```python
from build123d import *

# Parameters (mm, degrees)
SKETCH1_W                = 25
SKETCH1_H                = 25
BOSS_EXTRUDE1_DEPTH      = 5
SKETCH2_R                = 1.05
CUT_EXTRUDE1_DEPTH       = 5
FILLET1_R                = 2
SKETCH3_W                = 12
SKETCH3_H                = 12
SKETCH3_W_2              = 6
SKETCH3_H_2              = 6
BOSS_EXTRUDE2_DEPTH      = 98.425
SKETCH4_W                = 6
SKETCH4_H                = 6
CUT_EXTRUDE2_DEPTH       = 10
SKETCH5_W                = 12
SKETCH5_H                = 12
BOSS_EXTRUDE3_DEPTH      = 20
CUT_EXTRUDE3_DEPTH       = 20
CUT_EXTRUDE4_DEPTH       = 20
REVOLVE1_ANGLE           = 25
REVOLVE1_OTHER_WAY_ANGLE = 25


with BuildPart() as part:
    # Sketch1 → Boss-Extrude1 (new body)
    with BuildSketch(Plane(origin=(0, 0, 0), x_dir=(1, 0, 0), z_dir=(0, 1, 0))):
        with Locations((12.5, 12.5)):
            Rectangle(SKETCH1_W, SKETCH1_H)
    extrude(amount=BOSS_EXTRUDE1_DEPTH)

    # Sketch2 → Cut-Extrude1 (cut)
    with BuildSketch(Plane(origin=(0, 5, 0), x_dir=(1, 0, 0), z_dir=(0, 1, 0))):
        with Locations(Location((4.5, 4.5, 0), (0, 0, 270))):
            Circle(SKETCH2_R)
        with Locations(Location((20.5, 4.5, 0), (0, 0, 270))):
            Circle(SKETCH2_R)
        with Locations(Location((20.5, 20.5, 0), (0, 0, 270))):
            Circle(SKETCH2_R)
        with Locations(Location((4.5, 20.5, 0), (0, 0, 270))):
            Circle(SKETCH2_R)
    extrude(amount=-CUT_EXTRUDE1_DEPTH, mode=Mode.SUBTRACT)

    # Fillet1
    fillet1_edges = [part.edges().sort_by_distance(p)[0] for p in [
        (0, 2.5, -25),
        (25, 2.5, -25),
        (25, 2.5, 0),
        (0, 2.5, 0),
    ]]
    fillet(fillet1_edges, radius=FILLET1_R)

    # Sketch3 → Boss-Extrude2 (add)
    with BuildSketch(Plane(origin=(0, 5, 0), x_dir=(1, 0, 0), z_dir=(0, 1, 0))):
        with Locations((12.5, 12.5)):
            Rectangle(SKETCH3_W, SKETCH3_H)
        with Locations((12.5, 12.5)):
            Rectangle(SKETCH3_W_2, SKETCH3_H_2, mode=Mode.SUBTRACT)
    extrude(amount=BOSS_EXTRUDE2_DEPTH)

    # Sketch4 → Cut-Extrude2 (cut)
    with BuildSketch(Plane(origin=(0, 0, 0), x_dir=(-1, 0, 0), z_dir=(0, -1, 0))):
        with Locations((-12.5, 12.5)):
            Rectangle(SKETCH4_W, SKETCH4_H)
    extrude(amount=-CUT_EXTRUDE2_DEPTH, mode=Mode.SUBTRACT)

    # Sketch5 → Boss-Extrude3 (add)
    with BuildSketch(Plane(origin=(0, 103.425, 0), x_dir=(1, 0, 0), z_dir=(0, 1, 0))):
        with Locations((12.5, 12.5)):
            Rectangle(SKETCH5_W, SKETCH5_H)
    extrude(amount=BOSS_EXTRUDE3_DEPTH)

    # Sketch6 → Cut-Extrude3 (cut)
    with BuildSketch(Plane.XY.offset(-6.5)):
        Polygon((18.5, 123.425), (12.5, 123.425), (18.5, 103.425), align=None)
        Polygon((6.5, 103.425), (12.5, 123.425), (6.5, 123.425), align=None)
    extrude(amount=-CUT_EXTRUDE3_DEPTH, mode=Mode.SUBTRACT)

    # Sketch7 → Cut-Extrude4 (cut)
    with BuildSketch(Plane.ZY.offset(-6.5)):
        Polygon((-6.5, 123.425), (-6.5, 103.425), (-12.5, 123.425), align=None)
        Polygon((-18.5, 123.425), (-18.5, 103.425), (-12.5, 123.425), align=None)
    extrude(amount=-CUT_EXTRUDE4_DEPTH, mode=Mode.SUBTRACT)

    # Sketch8 → Revolve1 (revolve)
    with BuildSketch(Plane(origin=(12.5, 0, 0), x_dir=(0, 0, -1), z_dir=(1, 0, 0))):
        with BuildLine():
            ThreePointArc((24.627603923, 50.372343644), (16.394708904, 33.808356072), (20.558863125, 15.785979305))
            Line((20.558863125, 15.785979305), (22.064703847, 16.753815466))
            ThreePointArc((22.064703847, 16.753815466), (18.172495187, 33.599217247), (25.867730183, 49.081471856))
            Line((25.867730183, 49.081471856), (24.627603923, 50.372343644))
        make_face()
    revolve(axis=Axis((12.5, 54.79169199, -43.616981759), (0, -1, 0)), revolution_arc=REVOLVE1_ANGLE)

    # Sketch8 → Revolve1 other way (revolve)
    with BuildSketch(Plane(origin=(12.5, 0, 0), x_dir=(0, 0, -1), z_dir=(1, 0, 0))):
        with BuildLine():
            ThreePointArc((24.627603923, 50.372343644), (16.394708904, 33.808356072), (20.558863125, 15.785979305))
            Line((20.558863125, 15.785979305), (22.064703847, 16.753815466))
            ThreePointArc((22.064703847, 16.753815466), (18.172495187, 33.599217247), (25.867730183, 49.081471856))
            Line((25.867730183, 49.081471856), (24.627603923, 50.372343644))
        make_face()
    revolve(axis=Axis((12.5, 54.79169199, -43.616981759), (0, 1, 0)), revolution_arc=REVOLVE1_OTHER_WAY_ANGLE)


solid = part.part
```
Work out the finished part from the listing and answer in its coordinate system (mm). A direction names the side the tool comes from. Give positions to 0.01 mm unless a question says otherwise; leave off trailing zeros. Write each loop counter-clockwise with the first axis right and the second up, starting at its lowest first coordinate (ties: lowest second). Pieces come first, ordered by that corner, then holes.
(1) Flat-ended cylindrical pins translate along their axes: pin 1 Ø2.5 at (x, y) = (14, 3) entering from -Z; pin 2 Ø5 at (x, y) = (3, 105) entering from +Z; pin 3 Ø5 at (x, z) = (12, -5.5) entering from -Y; pin 4 Ø5 at (y, z) = (76.5, -19.5) entering from -X. Find the tip coordinate at first contact, or state that the pin passes through.
Final values:
pin 1: stops at z = -25
pin 2: passes through
pin 3: stops at y = 0
pin 4: stops at x = 6.5
(2) Which of the six approach directions +Z, -Z, +X, -X, +Y, -Y give full straight-line access (tool end or side, diameter ignored) to faces 1 (the flat face through (23.564, 33.16, -19.89)), 2 (the cylindrical face through (5.54, 2.54, -20.64)), 3 (the flat face through (1.436, 33.16, -19.89)), 4 (the conical face through (12.367, 16.599, -21.825)), 5 (the flat face through (7, 0, -13))?
Final values:
face 1: -Z, +X, +Y
face 2: -Y
face 3: -Z, -X, +Y
face 4: -Z
face 5: +Z, -Z, +X, -X, -Y
(3) The part is cut by section D-D on y = 18. Write down the section's boundary in (x, z).
Final values:
outline: (2.21, -21.56) - (3.07, -23.4) arc R22.3 cw to (21.93, -23.4) - (22.79, -21.56) arc R24.34 ccw to start; (6.5, -18.5) - (18.5, -18.5) - (18.5, -6.5) - (6.5, -6.5) - close; hole (9.5, -15.5) - (15.5, -15.5) - (15.5, -9.5) - (9.5, -9.5) - close
(4) The part is cut by section C-C on y = 75. Write down the section's boundary in (x, z), plus the area to 3 significant figures.
Final values:
outline: (6.5, -18.5) - (18.5, -18.5) - (18.5, -6.5) - (6.5, -6.5) - close; hole (9.5, -15.5) - (15.5, -15.5) - (15.5, -9.5) - (9.5, -9.5) - close
area: 108 mm2
(5) The mould has two halves that part along X. Classify faces 6 (the flat face through (12, 2, -25)), 7 (the conical face through (12.389, 49.449, -25.515)), 8 (the cylindrical face through (0.57, 2.54, -0.6)): pulls with the +X half, pulls with the -X half, needs draft (parallel to the pull), parting line crosses it, or undercut.
Final values:
face 6: needs draft
face 7: undercut
face 8: pulls with the -X half
(6) The part is cut by section A-A on z = -4.5. Write down the section's boundary in (x, y).
Final values:
outline: (0, 0) - (3.45, 0) - (3.45, 5) - (0, 5) - close; (5.55, 0) - (19.45, 0) - (19.45, 5) - (5.55, 5) - close; (21.55, 0) - (25, 0) - (25, 5) - (21.55, 5) - close
(7) Straight lines are drawn through the part: line 1 (X direction, y = 1, z = -20.5); line 2 (X direction, y = 16, z = -11); line 3 (Z direction, x = 15.25, y = 9.5). For each, find the intervals that lie inside material, in ascending order.
Final values:
line 1: x = 0 to 3.45, 5.55 to 19.45, 21.55 to 25
line 2: x = 6.5 to 9.5, 15.5 to 18.5
line 3: z = -18.5 to -15.5, -9.5 to -6.5
